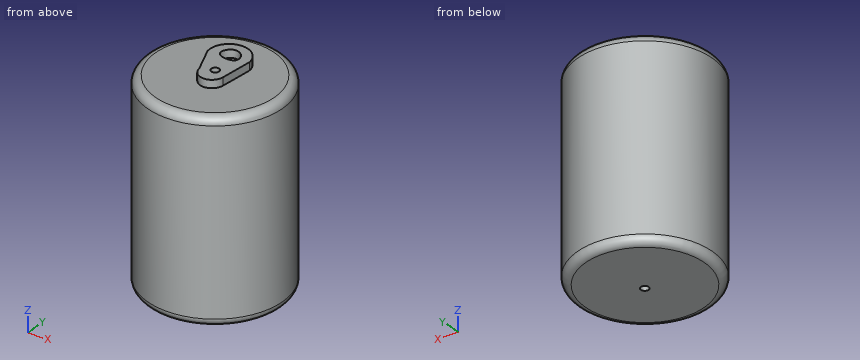
from build123d import *

# Parameters (mm, degrees)
F0_R     = 43.5266995613
F1_DEPTH = 127
F2_R     = 5.08
F4_DEPTH = 5.08
F6_DEPTH = 5.08
F8_D     = 5.08


with BuildPart() as f1:
    # F0 (on Top) → F1 (new body)
    with BuildSketch(Plane.XY):
        Circle(F0_R)
    extrude(amount=F1_DEPTH)

    # F2
    f2_edges = [f1.edges().sort_by_distance(p)[0] for p in [
        (43.5267, 0, 63.5),
        (-43.5267, 0, 0),
        (-43.5267, 0, 127),
    ]]
    fillet(f2_edges, radius=F2_R)

    # F3 (on face) → F4 (join)
    with BuildSketch(Plane.XY.offset(127)):
        with BuildLine():
            Line((9.7240488976, -6.4532333054), (11.8456594646, 14.0556711704))
            ThreePointArc((11.8456594646, 14.0556711704), (-2.1279540893, 25.2634606559), (-12.5528648496, 10.696454905))
            Line((-12.5528648496, 10.696454905), (-5.4808282293, -6.4532333054))
            ThreePointArc((-5.4808282293, -6.4532333054), (2.1216103341, -13.309783456), (9.7240488976, -6.4532333054))
        make_face()
    extrude(amount=F4_DEPTH)

    # F5 (on face) → F6 (cut)
    with BuildSketch(Plane.XY.offset(132.08)):
        with BuildLine():
            add(Edge.make_bspline(
                [(-5.6576291099, 12.0042935014), (-7.2494417271, 14.0385394216), (-4.3021102383, 20.9906666124), (4.4746239471, 19.4157133137), (7.4988739115, 8.9464331045), (-3.7704655796, 9.5926059252), (-5.6576291099, 12.0042935014)],
                knots=[0, 0, 0, 0, 0.2415357815, 0.4801991319, 0.7136487592, 1, 1, 1, 1], degree=3))
        make_face()
    extrude(amount=-F6_DEPTH, mode=Mode.SUBTRACT)

    # F8 (through all)
    with Locations(Plane.XY.offset(132.08)):
        with Locations((2.1216121968, -2.747733146)):
            Hole(F8_D / 2)


solid = f1.part
Here's how the part is built. I have some questions about the finished solid (model axes, mm). Round coordinates to 2 decimals unless told otherwise and drop trailing zeros. Write each loop counter-clockwise with the first axis right and the second up, starting at its lowest first coordinate (ties: lowest second). Pieces come first, ordered by that corner, then holes.
1. Will these pins go through, and if not, where does the flat tip stop? pin 1 Ø1.5 at (y, z) = (27, 113.5) entering from +X; pin 2 Ø10 at (y, z) = (-21.5, 50) entering from -X; pin 3 Ø6 at (x, z) = (20.5, 79.5) entering from +Y.
2. I need wall thicknesses on L1, parallel to Z at x = 28.5, y = 4; L2, parallel to X at y = -3, z = 105; L3, parallel to Y at x = 3, z = 66.5. Which ranges of each line are inside material? Lowest first, please.
3. Suppose I cut it at A-A (z = 59.5). List the corners of the cut face in (x, y) for me, and give its area (3 significant figures).
Answer sheet:
1. pin 1: stops at x = 34.72
1. pin 2: stops at x = -40.28
1. pin 3: stops at y = 39.85
2. L1: z = 0 to 127
2. L2: x = -43.42 to -0.41, 4.65 to 43.42
2. L3: y = -43.42 to -5.13, -0.36 to 43.42
3. outline: circle Ø87.05 at (0, 0); hole circle Ø5.08 at (2.12, -2.75)
3. area: 5,930 mm2
